CAD build for the part. Positions are in the model's coordinates, mm. Face numbers are marked on the shaded views. A direction names the side the tool comes from. Round coordinates to 2 decimals unless told otherwise and drop trailing zeros. Loops run counter-clockwise (first coordinate to the right, second up) from the corner with the lowest first, then second, coordinate; pieces in that order, holes last. Notation, with made-up numbers: M 13.25,66.25 L 42.25,66.25 A15 cw 42.25,95.25 Z; hole C -22,82 d1. An arc over 180 degrees is marked long. One line per item, written item: value. Start each with the question number.
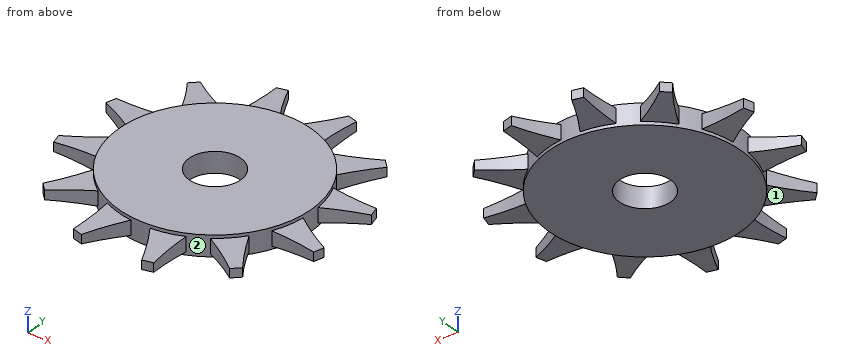
from build123d import *

# Parameters (mm, degrees)
BOSS_EXTRUDE1_DEPTH = 2
CUT_EXTRUDE1_DEPTH  = 2
CIRPATTERN1_COUNT   = 12
SKETCH6_R           = 9.317683155
SKETCH6_R_2         = 2.5
BOSS_EXTRUDE2_DEPTH = 2


with BuildPart() as part:
    # Sketch3 → Boss-Extrude1 (new body)
    with BuildSketch(Plane.XY):
        with BuildLine():
            Line((-7.563321911, 5.442001567), (-5.442001567, 7.563321911))
            add(Edge.make_bspline(
                [(-8.977535473, 9.684642254), (-7.300218474, 8.473386816), (-5.442001567, 7.563321911)],
                knots=[0, 0, 0, 1, 1, 1], degree=2))
            Line((-8.977535473, 9.684642254), (-9.684642254, 8.977535473))
            add(Edge.make_bspline(
                [(-9.684642254, 8.977535473), (-8.473386816, 7.300218474), (-7.563321911, 5.442001567)],
                knots=[0, 0, 0, 1, 1, 1], degree=2))
        make_face()
    extrude(amount=BOSS_EXTRUDE1_DEPTH)

    # Sketch4 → Cut-Extrude1 (cut, symmetric)
    with BuildSketch(Plane(origin=(0, 0, 0), x_dir=(0, 0, -1), z_dir=(-0.707106781186548, -0.7071067811865471, 0))):
        Polygon((0, -9.196152423), (-0.3, -9.196152423), (-0.6, -13.696152423), (0, -13.696152423), align=None)
        Polygon((-1.7, -9.196152423), (-2, -9.196152423), (-2, -13.696152423), (-1.4, -13.696152423), align=None)
    extrude(amount=CUT_EXTRUDE1_DEPTH, both=True, mode=Mode.SUBTRACT)


with BuildPart() as cirpattern1_1:
    # CirPattern1: pattern copy
    add(part.part.rotate(Axis((0, 0, 0), (0, 0, -1)), 1 * 360 / CIRPATTERN1_COUNT))


with BuildPart() as cirpattern1_2:
    # CirPattern1: pattern copy
    add(part.part.rotate(Axis((0, 0, 0), (0, 0, -1)), 2 * 360 / CIRPATTERN1_COUNT))


with BuildPart() as cirpattern1_3:
    # CirPattern1: pattern copy
    add(part.part.rotate(Axis((0, 0, 0), (0, 0, -1)), 3 * 360 / CIRPATTERN1_COUNT))


with BuildPart() as cirpattern1_4:
    # CirPattern1: pattern copy
    add(part.part.rotate(Axis((0, 0, 0), (0, 0, -1)), 4 * 360 / CIRPATTERN1_COUNT))


with BuildPart() as cirpattern1_5:
    # CirPattern1: pattern copy
    add(part.part.rotate(Axis((0, 0, 0), (0, 0, -1)), 5 * 360 / CIRPATTERN1_COUNT))


with BuildPart() as cirpattern1_6:
    # CirPattern1: pattern copy
    add(part.part.rotate(Axis((0, 0, 0), (0, 0, -1)), 6 * 360 / CIRPATTERN1_COUNT))


with BuildPart() as cirpattern1_7:
    # CirPattern1: pattern copy
    add(part.part.rotate(Axis((0, 0, 0), (0, 0, -1)), 7 * 360 / CIRPATTERN1_COUNT))


with BuildPart() as cirpattern1_8:
    # CirPattern1: pattern copy
    add(part.part.rotate(Axis((0, 0, 0), (0, 0, -1)), 8 * 360 / CIRPATTERN1_COUNT))


with BuildPart() as cirpattern1_9:
    # CirPattern1: pattern copy
    add(part.part.rotate(Axis((0, 0, 0), (0, 0, -1)), 9 * 360 / CIRPATTERN1_COUNT))


with BuildPart() as cirpattern1_10:
    # CirPattern1: pattern copy
    add(part.part.rotate(Axis((0, 0, 0), (0, 0, -1)), 10 * 360 / CIRPATTERN1_COUNT))


with BuildPart() as cirpattern1_11:
    # CirPattern1: pattern copy
    add(part.part.rotate(Axis((0, 0, 0), (0, 0, -1)), 11 * 360 / CIRPATTERN1_COUNT))


with BuildPart() as part_1:
    add(part.part)

    add(cirpattern1_1.part)  # Boss-Extrude2 merges CirPattern1_1

    add(cirpattern1_2.part)  # Boss-Extrude2 merges CirPattern1_2

    add(cirpattern1_3.part)  # Boss-Extrude2 merges CirPattern1_3

    add(cirpattern1_4.part)  # Boss-Extrude2 merges CirPattern1_4

    add(cirpattern1_5.part)  # Boss-Extrude2 merges CirPattern1_5

    add(cirpattern1_6.part)  # Boss-Extrude2 merges CirPattern1_6

    add(cirpattern1_7.part)  # Boss-Extrude2 merges CirPattern1_7

    add(cirpattern1_8.part)  # Boss-Extrude2 merges CirPattern1_8

    add(cirpattern1_9.part)  # Boss-Extrude2 merges CirPattern1_9

    add(cirpattern1_10.part)  # Boss-Extrude2 merges CirPattern1_10

    add(cirpattern1_11.part)  # Boss-Extrude2 merges CirPattern1_11
    # Sketch6 → Boss-Extrude2 (add)
    with BuildSketch(Plane.XY):
        Circle(SKETCH6_R)
        Circle(SKETCH6_R_2, mode=Mode.SUBTRACT)
    extrude(amount=BOSS_EXTRUDE2_DEPTH)


solid = part_1.part
(1) Slice it at A-A, the plane x = 0. List the corners of the cut face in (y, z).
(2) Slice it at C-C, the plane y = 5. List the corners of the cut face in (x, z), and give its area (4 significant figures).
(3) Flat gauge pins, fed straight in: P1, Ø12, axis at x = 1.5, y = 3, coming from the -Z side; P2, Ø4, axis at x = 0, y = 0, coming from the -Z side. Where does each tip first touch, or does it go through?
(4) Which spindle directions (+Z, -Z, +X, -X, +Y, -Y) get a long thin tool onto all of the face, cutting with end or side? Do the marked faces 1 and 2. Say none if no direction does.
(5) Probe L1, parallel to Y at x = 0, z = 1.25; L2, parallel to X at y = -8.75, z = 1.35; L3, parallel to Y at x = 0.5, z = 1.95. List the from-to ranges inside material, lowest first.
Check result:
1. outline: M -9.32,0 L -2.5,0 L -2.5,2 L -9.32,2 Z; M 2.5,0 L 9.32,0 L 9.32,2 L 2.5,2 Z
2. outline: M -7.86,0 L 7.86,0 L 7.86,2 L -7.86,2 Z
2. area: 31.45 mm^2
3. P1: stops at z = 0
3. P2: passes through
4. face 1: -Z, -X, -Y
4. face 2: none
5. L1: y = -9.32 to -2.5, 2.5 to 9.32
5. L2: x = -9.52 to -7.58, -3.81 to 3.81, 7.58 to 9.52
5. L3: y = -9.3 to -2.45, 2.45 to 9.3
